from build123d import *

# Parameters (mm, degrees)
SKETCH_W     = 64
SKETCH_H     = 5
PAD_DEPTH    = 2
SKETCH001_W  = 3
SKETCH001_H  = 5
PAD001_DEPTH = 5.5
SKETCH002_R  = 0.75
POCKET_DEPTH = 70
SKETCH003_W  = 3
SKETCH003_H  = 5
PAD002_DEPTH = 10
FILLET_R     = 2.49


with BuildPart() as part:
    # Sketch → Pad (new body)
    with BuildSketch(Plane.XY):
        Rectangle(SKETCH_W, SKETCH_H)
    extrude(amount=PAD_DEPTH)

    # Sketch001 (on Face6 of Pad) → Pad001 (join)
    with BuildSketch(Plane.XY.offset(2)):
        with Locations((-27.3, 0)):
            Rectangle(SKETCH001_W, SKETCH001_H)
        with Locations((27.3, 0)):
            Rectangle(SKETCH001_W, SKETCH001_H)
    extrude(amount=PAD001_DEPTH)

    # Sketch002 (on Face15 of Pad001) → Pocket (cut)
    with BuildSketch(Plane.YZ.offset(28.8)):
        with Locations((0, 5)):
            Circle(SKETCH002_R)
    extrude(amount=-POCKET_DEPTH, mode=Mode.SUBTRACT)

    # Sketch003 (on Face4 of Pocket) → Pad002 (join)
    with BuildSketch(Plane(origin=(0, 0, 0), x_dir=(1, 0, 0), z_dir=(0, 0, -1))):
        with Locations((-27.3, 0)):
            Rectangle(SKETCH003_W, SKETCH003_H)
        with Locations((27.3, 0)):
            Rectangle(SKETCH003_W, SKETCH003_H)
    extrude(amount=PAD002_DEPTH)

    # Fillet
    fillet_edges = [part.edges().sort_by_distance(p)[0] for p in [
        (27.3, -2.5, 7.5),
        (-27.3, -2.5, 7.5),
        (-27.3, 2.5, 7.5),
        (27.3, 2.5, 7.5),
    ]]
    fillet(fillet_edges, radius=FILLET_R)


solid = part.part
Source: CAD feature listing. Evaluate the final solid. Frame: model axes, mm. A direction names the side the tool comes from. Coordinates: 2 decimals unless noted, no trailing zeros. Loops run counter-clockwise (first coordinate to the right, second up) from the corner with the lowest first, then second, coordinate; pieces in that order, holes last. Notation, with made-up numbers: (-8.5, 34) - (0.5, 34) arc R32 ccw to (0.5, 70) - close; hole circle Ø5 at (85, 71.5). An arc over 180 degrees is marked (long way). One line per item, written item: value. Start each with the question number.
1. Section A-A (z = -9). Return the cut outline in (x, y), and give its area (3 significant figures).
2. Section B-B (x = -24). Return the cut outline in (y, z), and give its area (3 significant figures).
3. Contact query for flat-ended pins moving along their axis: P1, Ø2.5, axis at x = 8.5, y = -1, coming from the +Z side; P2, Ø1.5, axis at y = 1, z = -5.5, coming from the -X side; P3, Ø3, axis at x = -5, y = -1, coming from the -Z side. Output: stop coordinate, or through.
4. Ray query, L1, parallel to X at y = -0.5, z = -6.5; L2, parallel to Z at x = 27.05, y = 0; L3, parallel to Z at x = 16.5, y = 1.15. Return the intervals inside material, ascending.
5. Mould query, pull axis Y, two halves, no side actions, for faces 4 (the cylindrical face through (27.321, -0.163, 4.268)), 5 (the flat face through (27, 0, -10)), 6 (the flat face through (0, -2.5, 1)). Classes: pulls with the +Y half, pulls with the -Y half, needs draft (parallel to the pull), parting line crosses it, or undercut.
6. Set-up query: faces 1 (the flat face through (-25.8, 0, -5)), 2 (the flat face through (-28.8, 0, 4)), 3 (the flat face through (30, 0, 0)). Return all of +Z, -Z, +X, -X, +Y, -Y with unobstructed straight access to the full face (end or side cutting, diameter ignored); none if empty.
Verdict:
1. outline: (-28.8, -2.5) - (-25.8, -2.5) - (-25.8, 2.5) - (-28.8, 2.5) - close; (25.8, -2.5) - (28.8, -2.5) - (28.8, 2.5) - (25.8, 2.5) - close
1. area: 30.0 mm2
2. outline: (-2.5, 0) - (2.5, 0) - (2.5, 2) - (-2.5, 2) - close
2. area: 10.0 mm2
3. P1: stops at z = 2
3. P2: stops at x = -28.8
3. P3: stops at z = 0
4. L1: x = -28.8 to -25.8, 25.8 to 28.8
4. L2: z = -10 to 4.25, 5.75 to 7.5
4. L3: z = 0 to 2
5. face 4: undercut
5. face 5: needs draft
5. face 6: pulls with the -Y half
6. face 1: -Z, +Y, -Y
6. face 2: +Z, -X, +Y, -Y
6. face 3: -Z, +X, +Y, -Y
